For this review, take the finished solid that the model builds, in its own axes (mm). Give positions to 0.01 mm unless a question says otherwise; leave off trailing zeros. Write each loop counter-clockwise with the first axis right and the second up, starting at its lowest first coordinate (ties: lowest second). Pieces come first, ordered by that corner, then holes.
1) We need section B-B on x = 20. Give the boundary of the cut face in (y, z), and give its area (3 significant figures).
2) We need section A-A on y = -16.5. Give the boundary of the cut face in (x, z), and give its area (3 significant figures).
3) We need section C-C on z = 0.8. Give the boundary of the cut face in (x, y) (1 decimal).
4) For P1, Ø0.8, axis at y = 3.5, z = 1.5, coming from the -X side; P2, Ø1.2, axis at x = -17, z = 1, coming from the +Y side; P3, Ø0.8, axis at y = 4, z = 1.5, coming from the +X side, all flat-tipped, find the tip position at first contact; note any pin that passes through.
5) Wall thickness on line 1 along X through (y, z) = (-0.5, 0.7); line 2 along X through (y, z) = (4.5, 1.7); line 3 along X through (y, z) = (-20, 1.25): over which ranges is each line inside the solid? List them lowest first.
6) We need section D-D on y = 3. Give the boundary of the cut face in (x, z).
Autodesk Inventor part; units mm, degrees
ref_plane "Work Plane1" through (0, -15.9764, 0) normal (-1, 0, 0) x (0, 0, 1)
ref_plane "YZ Plane" through (0, 0, 0) normal (1, 0, 0) x (0, 1, 0)
ref_plane "XZ Plane" through (0, 0, 0) normal (0, 1, 0) x (-1, 0, 0)
sketch "Sketch1" plane through (0, 0, 0) normal (0, 0, 1) x (1, 0, 0)
  circle A0 centre (0, -15.9764) radius 16 construction
  line L0 (-3, 0.0236) -> (0, 0.0236) construction
  line L1 (-3.206, 0) -> (3.4858, 0)
  line L2 (-13.7477, -21.9764) -> (13.7477, -21.9764) construction
  arc A1 (-14.2074, -11.165) -> (-13.7477, -21.9764) centre (0, -15.9764) ccw
  line L3 (0, 1.949) -> (0, -3.4788)
  arc A2 (-3, 2.0236) -> (3, 2.0236) centre (0, 2.0236) ccw
  arc A3 (23.9912, -26.7519) -> (-23.9912, -26.7519) centre (0, -15.9764) ccw
  line L4 (-18, -9.9764) -> (-15.0599, -9.9764)
  line L5 (-3, 2.0236) -> (-3, 4.9378)
  arc A4 (-6, 7.2615) -> (-21.1765, -4.6822) centre (0, -15.9764) ccw
  arc A5 (-3, 4.9378) -> (-6, 7.2615) centre (-5.4, 4.9378) ccw
  arc A6 (-21.1765, -4.6822) -> (-18, -9.9764) centre (-18, -6.3764) ccw
  arc A7 (-14.2074, -11.165) -> (-15.0599, -9.9764) centre (-15.0599, -10.8764) ccw
  line L6 (0, 10.3236) -> (2.5298, 10.3236) construction
  line L7 (-13.7477, -21.9764) -> (-15.7457, -26.6705)
  arc A8 (-23.9912, -26.7519) -> (-15.7457, -26.6705) centre (-19.8862, -24.9082) ccw
  line L8 (0, -0.9764) -> (-1.2778, -0.9764) construction
  line L9 (13.7477, -21.9764) -> (15.7457, -26.6705)
  arc A9 (15.7457, -26.6705) -> (23.9912, -26.7519) centre (19.8862, -24.9082) ccw
  arc A10 (13.7477, -21.9764) -> (14.2074, -11.165) centre (0, -15.9764) ccw
  line L10 (18, -9.9764) -> (15.0599, -9.9764)
  line L11 (3, 2.0236) -> (3, 4.9378)
  arc A11 (21.1765, -4.6822) -> (6, 7.2615) centre (0, -15.9764) ccw
  arc A12 (6, 7.2615) -> (3, 4.9378) centre (5.4, 4.9378) ccw
  arc A13 (18, -9.9764) -> (21.1765, -4.6822) centre (18, -6.3764) ccw
  arc A14 (15.0599, -9.9764) -> (14.2074, -11.165) centre (15.0599, -10.8764) ccw
  point P0 (3, 0.0236)
  dimension "d0" = 32
  dimension "d3" = 6
  dimension "d4" = 3
  dimension "d5" = 52.6
  dimension "d8" = 24
  dimension "d9" = 6
  dimension "d10" = 2.4
  dimension "d11" = 3.6
  dimension "d12" = 0.9
  dimension "d13" = 4.5
  dimension "d14" = 15
  dimension "d15" = 15
extrude "Body" add sketch "Sketch1" along normal blind 2.5
ref_plane "Work Plane1" through (0, -15.9764, 0) normal (-1, 0, 0) x (0, 0, 1)
equation "\"d0\" = WD"
equation "\"d3\" = 0.2 * ND"
equation "\"d4\" = 0.1 * ND"
equation "\"d5\" = SD2"
equation "\"d8\" = 0.8 * ND"
equation "\"d9\" = 0.2 * ND"
equation "\"d10\" = 0.08 * ND"
equation "\"d11\" = 0.12 * ND"
equation "\"d12\" = 0.03 * ND"
equation "\"d13\" = 0.15 * ND"
equation "\"d14\" = 0.5 * ND"
equation "\"d15\" = 0.5 * ND"
equation "\"d16\" = SD"
equation "\"SD\" = 2.5"
equation "\"WD\" = 32"
equation "\"d1\" = 1.6 * ND"
equation "\"SD2\" = 52.6"
equation "\"d7\" = 0.15 * ND"
equation "\"WDMIN\" = 25"
equation "\"SNB\" = 2.55"
equation "\"WDMAX\" = 38"
equation "\"BUBRMI\" = 4"
properties part number "DIN 6799 - 30" material "Steel, Mild"
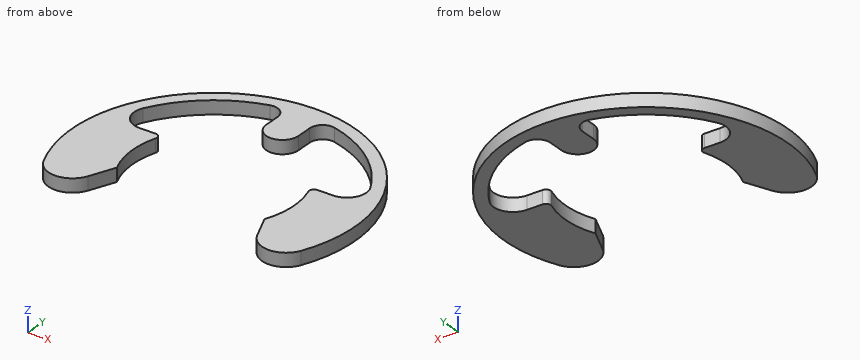
Results list:
1. outline: (-29.41, 0) - (-9.37, 0) - (-9.37, 2.5) - (-29.41, 2.5) - close; (-2.71, 0) - (1.1, 0) - (1.1, 2.5) - (-2.71, 2.5) - close
1. area: 59.6 mm2
2. outline: (-26.29, 0) - (-14.99, 0) - (-14.99, 2.5) - (-26.29, 2.5) - close; (14.99, 0) - (26.29, 0) - (26.29, 2.5) - (14.99, 2.5) - close
2. area: 56.5 mm2
3. outline: (-24, -26.8) arc R4.5 ccw to (-15.7, -26.7) - (-13.7, -22) arc R15 cw to (-14.2, -11.2) arc R0.9 ccw to (-15.1, -10) - (-18, -10) arc R3.6 cw to (-21.2, -4.7) arc R24 cw to (-6, 7.3) arc R2.4 cw to (-3, 4.9) - (-3, 2) arc R3 ccw to (3, 2) - (3, 4.9) arc R2.4 cw to (6, 7.3) arc R24 cw to (21.2, -4.7) arc R3.6 cw to (18, -10) - (15.1, -10) arc R0.9 ccw to (14.2, -11.2) arc R15 cw to (13.7, -22) - (15.7, -26.7) arc R4.5 ccw to (24, -26.8) arc R26.3 ccw (long way) to start
4. P1: stops at x = -18.1
4. P2: stops at y = 4.58
4. P3: stops at x = 17.56
5. line 1: x = -21.26 to -18.34, -1.62 to 1.62, 18.34 to 21.26
5. line 2: x = -16.5 to -12.52, -3 to 3, 12.52 to 16.5
5. line 3: x = -25.99 to -14.45, 14.45 to 25.99
6. outline: (-18.21, 0) - (-14.69, 0) - (-14.69, 2.5) - (-18.21, 2.5) - close; (-3, 0) - (3, 0) - (3, 2.5) - (-3, 2.5) - close; (14.69, 0) - (18.21, 0) - (18.21, 2.5) - (14.69, 2.5) - close
